The model under review builds one solid part; all positions refer to its coordinate system, in mm. A direction names the side the tool comes from. Give positions to 0.01 mm unless a question says otherwise; leave off trailing zeros. Order: outer loops, then holes, each group sorted by start corner. A loop starts at its lowest first (then second) coordinate and runs counter-clockwise, first axis right, second up. Notation, with made-up numbers: (-30, 57) -> (25, 57) arc R16 ccw to (25, 61) -> close; hole circle Ø2 at (-35.5, -29). An arc over 180 degrees is marked (long way). Answer as a JSON object with one key per item and string values. Group by question number.
from build123d import *

# Parameters (mm, degrees)
F0_R     = 5.75
F0_R_2   = 3.75
F1_DEPTH = 11
F2_W     = 24
F2_H     = 12
F2_R     = 5.75
F3_DEPTH = 2
F4_D     = 3
F5_R     = 5.99999


# Not quite as in the source:
# - a fillet or chamfer is up to 0.001 mm smaller than in the source, because OpenCascade refuses the exact size


with BuildPart() as f1:
    # F0 (on Front) → F1 (new body)
    with BuildSketch(Plane.XZ):
        Circle(F0_R)
        Circle(F0_R_2, mode=Mode.SUBTRACT)
    extrude(amount=F1_DEPTH)

    # F2 (on face) → F3 (join)
    with BuildSketch(Plane.XZ.offset(11)):
        Rectangle(F2_W, F2_H)
        Circle(F2_R, mode=Mode.SUBTRACT)
    extrude(amount=-F3_DEPTH)

    # F4 (through all)
    with Locations(Plane.XZ.offset(11)):
        with Locations((-8.75, 0), (8.75, 0)):
            Hole(F4_D / 2)

    # F5 (radius 6 in the source; OpenCascade refuses exactly that, so slightly less here)
    f5_edges = [f1.edges().sort_by_distance(p)[0] for p in [
        (12, -10, 6),
        (12, -10, -6),
        (-12, -10, 6),
        (-12, -10, -6),
    ]]
    fillet(f5_edges, radius=F5_R)


solid = f1.part
1. Machinability: for faces 5 (the cylindrical face through (-0.75, -4.44, 5.7)), 6 (the cylindrical face through (-3.746, -5.423, 0.165)), which of the approach directions +Z, -Z, +X, -X, +Y, -Y give a long, thin tool a straight path to every point of the face, cutting with its end or side? Answer none if there is none.
2. Take a section at C-C on z = 1. Give the boundary of the cut face in (x, y).
3. For pin 1 (5 mm diameter, centred on x = 3, y = -3, fed in from +Z); pin 2 (2.5 mm diameter, centred on x = 8.75, z = 0, fed in from +Y); pin 3 (6 mm diameter, centred on x = -2, y = -1.5, fed in from -Z); pin 4 (4 mm diameter, centred on y = -2.5, z = -0.5, fed in from +X), all flat-tipped, find the tip position at first contact; note any pin that passes through.
4. Take a section at B-B on z = 2.25. Give the boundary of the cut face in (x, y).
5. Take a section at D-D on y = -5.5. Give the boundary of the cut face in (x, z).
6. Take a section at A-A on x = 0. Give the boundary of the cut face in (y, z), plus the area to 3 significant figures.
7. For probe 1 along Z at (x, y) = (0, -8.5); probe 2 along Y at (x, z) = (-7, 1.25); probe 3 along X at (y, z) = (-1.5, 1.5), list the stretches that pass through material, from the lowest coordinate up. Write a range as [from, to].
8. Draft analysis for pull direction Z (two halves, no side actions). For faces 1 (the flat face through (5.2, -9, 2.8)), 2 (the cylindrical face through (-7.56, -9.99, -0.91)), 3 (the cylindrical face through (10.196, -9.986, 4.289)), 4 (the cylindrical face through (-10.289, -9.986, -4.196)), state which applies: pulls with the +Z half, pulls with the -Z half, needs draft (parallel to the pull), parting line crosses it, or undercut.
Checks:
{
 "1": {"face 5": "+Y", "face 6": "+Y, -Y"},
 "2": {"outline": "(-11.92, -11) -> (-9.87, -11) -> (-9.87, -9) -> (-11.92, -9) -> close; (-7.63, -11) -> (-3.61, -11) -> (-3.61, 0) -> (-5.66, 0) -> (-5.66, -9) -> (-7.63, -9) -> close; (3.61, -11) -> (7.63, -11) -> (7.63, -9) -> (5.66, -9) -> (5.66, 0) -> (3.61, 0) -> close; (9.87, -11) -> (11.92, -11) -> (11.92, -9) -> (9.87, -9) -> close"},
 "3": {"pin 1": "stops at z = 5.73", "pin 2": "passes through", "pin 3": "stops at z = -5.75", "pin 4": "stops at x = 5.75"},
 "4": {"outline": "(-11.56, -11) -> (-3, -11) -> (-3, 0) -> (-5.29, 0) -> (-5.29, -9) -> (-11.56, -9) -> close; (3, -11) -> (11.56, -11) -> (11.56, -9) -> (5.29, -9) -> (5.29, 0) -> (3, 0) -> close"},
 "5": {"outline": "circle Ø11.5 at (0, 0); hole circle Ø7.5 at (0, 0)"},
 "6": {"outline": "(-11, -6) -> (-9, -6) -> (-9, -5.75) -> (0, -5.75) -> (0, -3.75) -> (-11, -3.75) -> close; (-11, 3.75) -> (0, 3.75) -> (0, 5.75) -> (-9, 5.75) -> (-9, 6) -> (-11, 6) -> close", "area": "45.0 mm2"},
 "7": {"probe 1": "z = [-5.75, -3.75], [3.75, 5.75]", "probe 2": "y = [-11, -9]", "probe 3": "x = [-5.55, -3.44], [3.44, 5.55]"},
 "8": {"face 1": "needs draft", "face 2": "undercut", "face 3": "pulls with the +Z half", "face 4": "pulls with the -Z half"}
}
